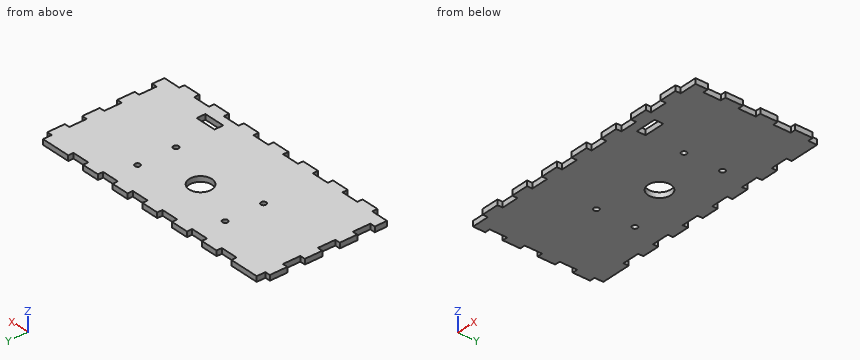
```python
from build123d import *

# Parameters (mm, degrees)
MDFESB_W          = 150
MDFESB_H          = 75
MDF_DEPTH         = 3
ENCAIXESESB_W     = 10
ENCAIXESESB_H     = 3
ENCAIXESESB_W_2   = 3
ENCAIXESESB_H_2   = 10
ENCAIXES_DEPTH    = 3
MOTORPASSOESB_R   = 1.5
MOTORPASSOESB_R_2 = 6.5
MOTORPASSOESB_W   = 12
MOTORPASSOESB_H   = 5
MOTORPASSO_DEPTH  = 3


with BuildPart() as part:
    # mdfEsb → mdf (new body)
    with BuildSketch(Plane.XY):
        with Locations((75, 37.5)):
            Rectangle(MDFESB_W, MDFESB_H)
    extrude(amount=MDF_DEPTH)

    # EncaixesEsb → Encaixes (cut)
    with BuildSketch(Plane.XY.offset(3)):
        with Locations((25, 1.5)):
            Rectangle(ENCAIXESESB_W, ENCAIXESESB_H)
        with Locations((5, 1.5)):
            Rectangle(ENCAIXESESB_W, ENCAIXESESB_H)
        with Locations((45, 1.5)):
            Rectangle(ENCAIXESESB_W, ENCAIXESESB_H)
        with Locations((65, 1.5)):
            Rectangle(ENCAIXESESB_W, ENCAIXESESB_H)
        with Locations((85, 1.5)):
            Rectangle(ENCAIXESESB_W, ENCAIXESESB_H)
        with Locations((105, 1.5)):
            Rectangle(ENCAIXESESB_W, ENCAIXESESB_H)
        with Locations((125, 1.5)):
            Rectangle(ENCAIXESESB_W, ENCAIXESESB_H)
        with Locations((145, 1.5)):
            Rectangle(ENCAIXESESB_W, ENCAIXESESB_H)
        with Locations((1.5, 15)):
            Rectangle(ENCAIXESESB_W_2, ENCAIXESESB_H_2)
        with Locations((148.5, 15)):
            Rectangle(ENCAIXESESB_W_2, ENCAIXESESB_H_2)
        with Locations((148.5, 35)):
            Rectangle(ENCAIXESESB_W_2, ENCAIXESESB_H_2)
        with Locations((148.5, 55)):
            Rectangle(ENCAIXESESB_W_2, ENCAIXESESB_H_2)
        with Locations((148.5, 75)):
            Rectangle(ENCAIXESESB_W_2, ENCAIXESESB_H_2)
        with Locations((1.5, 35)):
            Rectangle(ENCAIXESESB_W_2, ENCAIXESESB_H_2)
        with Locations((1.5, 55)):
            Rectangle(ENCAIXESESB_W_2, ENCAIXESESB_H_2)
        with Locations((1.5, 75)):
            Rectangle(ENCAIXESESB_W_2, ENCAIXESESB_H_2)
        with Locations((25, 73.5)):
            Rectangle(ENCAIXESESB_W, ENCAIXESESB_H)
        with Locations((45, 73.5)):
            Rectangle(ENCAIXESESB_W, ENCAIXESESB_H)
        with Locations((65, 73.5)):
            Rectangle(ENCAIXESESB_W, ENCAIXESESB_H)
        with Locations((85, 73.5)):
            Rectangle(ENCAIXESESB_W, ENCAIXESESB_H)
        with Locations((105, 73.5)):
            Rectangle(ENCAIXESESB_W, ENCAIXESESB_H)
        with Locations((125, 73.5)):
            Rectangle(ENCAIXESESB_W, ENCAIXESESB_H)
    extrude(amount=-ENCAIXES_DEPTH, mode=Mode.SUBTRACT)

    # motorPassoEsb → motorPasso (cut)
    with BuildSketch(Plane.XY.offset(3)):
        with Locations((45.5, 35)):
            Circle(MOTORPASSOESB_R)
        with Locations((104.5, 35)):
            Circle(MOTORPASSOESB_R)
        with Locations((104.5, 57)):
            Circle(MOTORPASSOESB_R)
        with Locations((45.5, 57)):
            Circle(MOTORPASSOESB_R)
        with Locations((75, 46)):
            Circle(MOTORPASSOESB_R_2)
        with Locations((110.5, 10.5)):
            Rectangle(MOTORPASSOESB_W, MOTORPASSOESB_H)
    extrude(amount=-MOTORPASSO_DEPTH, mode=Mode.SUBTRACT)


solid = part.part
```
CAD build for the part. Positions are in the model's coordinates, mm. Round coordinates to 2 decimals unless told otherwise and drop trailing zeros. Order: outer loops, then holes, each group sorted by start corner. A loop starts at its lowest first (then second) coordinate and runs counter-clockwise, first axis right, second up. Notation, with made-up numbers: (31.5, -36.5) - (61.5, -36.5) arc R30 ccw to (61.5, -14.5) - close; hole circle Ø8 at (38.5, 33). An arc over 180 degrees is marked (long way). Answer in a Markdown table with one row per item. Add a question column.
(1) Band-saw the part on C-C on x = 45.5. List the corners of the cut face in (y, z).
(2) Band-saw the part on A-A on y = 46. List the corners of the cut face in (x, z).
(3) Drop flat-ended pins along their axis: pin 1 Ø0.9 at (x, z) = (87.5, 1) entering from -Y; pin 2 Ø1.5 at (y, z) = (1.5, 1.5) entering from +X; pin 3 Ø0.9 at (y, z) = (73, 2) entering from -X. Give the stop position or say it passes through.
(4) Band-saw the part on B-B on x = 75. List the corners of the cut face in (y, z).
(5) Band-saw the part on D-D on y = 35. List the corners of the cut face in (x, z), and give its area (3 significant figures).
(6) Probe L1, parallel to Y at x = 45.5, z = 0.8; L2, parallel to X at y = 9.5, z = 1.3; L3, parallel to Y at x = 109, z = 0.35. List the from-to ranges inside material, lowest first. Write a range as [from, to].
Data:
| question | item | result |
|---|---|---|
| 1 | outline | (3, 0) - (33.5, 0) - (33.5, 3) - (3, 3) - close; (36.5, 0) - (55.5, 0) - (55.5, 3) - (36.5, 3) - close; (58.5, 0) - (72, 0) - (72, 3) - (58.5, 3) - close |
| 2 | outline | (0, 0) - (68.5, 0) - (68.5, 3) - (0, 3) - close; (81.5, 0) - (150, 0) - (150, 3) - (81.5, 3) - close |
| 3 | pin 1 | stops at y = 3 |
| 3 | pin 2 | stops at x = 140 |
| 3 | pin 3 | stops at x = 3 |
| 4 | outline | (0, 0) - (39.5, 0) - (39.5, 3) - (0, 3) - close; (52.5, 0) - (75, 0) - (75, 3) - (52.5, 3) - close |
| 5 | outline | (3, 0) - (44, 0) - (44, 3) - (3, 3) - close; (47, 0) - (103, 0) - (103, 3) - (47, 3) - close; (106, 0) - (147, 0) - (147, 3) - (106, 3) - close |
| 5 | area | 414 mm^2 |
| 6 | L1 | y = [3, 33.5], [36.5, 55.5], [58.5, 72] |
| 6 | L2 | x = [0, 104.5], [116.5, 150] |
| 6 | L3 | y = [3, 8], [13, 72] |
